Input: dimensioned drawing with shaded views. Units: mm. Origin: part minimum x, y, z. A direction names the side the tool comes from. Round coordinates to 2 decimals unless told otherwise and drop trailing zeros. Order: outer loops, then holes, each group sorted by start corner. A loop starts at its lowest first (then second) coordinate and runs counter-clockwise, first axis right, second up. Notation, with made-up numbers: (62, 36.25) - (75, 36.25) arc R23 cw to (75, 64.25) - close; hole circle Ø1 at (25, -18). An arc over 180 degrees is marked (long way). Return JSON: item names as keys, results as strings. Group by question number.
1) Contact query for flat-ended pins moving along their axis: P1, Ø2, axis at y = 7.5, z = 3.5, coming from the -X side; P2, Ø3, axis at x = 2.5, y = 11.5, coming from the +Z side; P3, Ø3, axis at x = 10, y = 4.5, coming from the +Z side. Output: stop coordinate, or through.
2) Section D-D, the plane z = 1.5. Return loops of the section in (x, y), plus the area to 3 significant figures.
3) Section A-A, the plane x = 6.5. Return loops of the section in (y, z), plus the area to 3 significant figures.
4) Ray query, line 1 (Z direction, x = 2.5, y = 6); line 2 (Z direction, x = 9.25, y = 5); line 3 (Y direction, x = 7.75, z = 1.35). Return the intervals inside material, ascending. Write a range as from..to.
5) Access query for the marked faces 1 and 2. Directions: +Z, -Z, +X, -X, +Y, -Y. A direction counts if a zero-diameter tool reaches every point of the face in a straight line with its end or side. Return the directions, or none.
6) Section C-C, the plane z = 3.6. Return loops of the section in (x, y), plus the area to 3 significant figures.
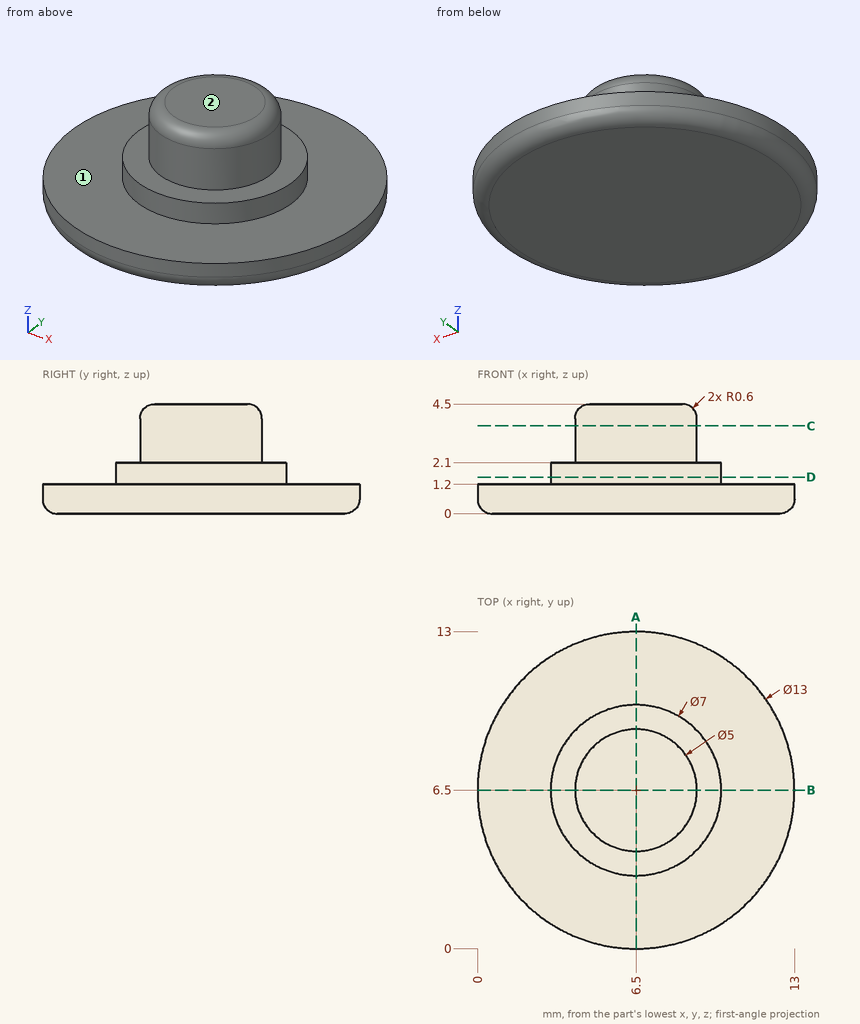
Geometry check:
{
 "1": {"P1": "x = 4", "P2": "z = 1.2", "P3": "z = 2.1"},
 "2": {"outline": "circle Ø7 at (6.5, 6.5)", "area": "38.5 mm2"},
 "3": {"outline": "(0, 0.6) arc R0.6 ccw to (0.6, 0) - (12.4, 0) arc R0.6 ccw to (13, 0.6) - (13, 1.2) - (10, 1.2) - (10, 2.1) - (9, 2.1) - (9, 3.9) arc R0.6 ccw to (8.4, 4.5) - (4.6, 4.5) arc R0.6 ccw to (4, 3.9) - (4, 2.1) - (3, 2.1) - (3, 1.2) - (0, 1.2) - close", "area": "33.6 mm2"},
 "4": {"line 1": "0..1.2", "line 2": "0..2.1", "line 3": "3.23..9.77"},
 "5": {"face 1": "+Z", "face 2": "+Z, +X, -X, +Y, -Y"},
 "6": {"outline": "circle Ø5 at (6.5, 6.5)", "area": "19.6 mm2"}
}
